Could you check a few things on this drawing? It's one solid part, dimensions in mm from its lowest x, y, z. Round coordinates to 2 decimals unless told otherwise and drop trailing zeros. Order: outer loops, then holes, each group sorted by start corner. A loop starts at its lowest first (then second) coordinate and runs counter-clockwise, first axis right, second up. Notation, with made-up numbers: (74, -12) - (79, -12) arc R27 ccw to (79, 6) - close; hole circle Ø1 at (61.5, 69.25). An arc over 180 degrees is marked (long way). Use one line per item in the form item = value.
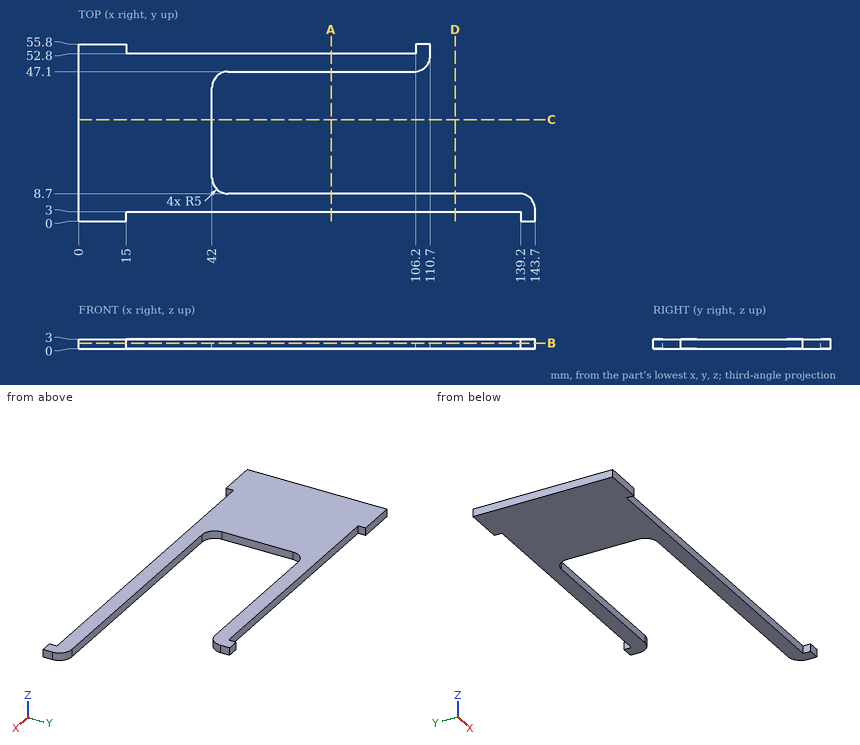
Item 1: Imagine slicing it at B-B on z = 1.8. Please give me the cut outline in (x, y), plus the area to 3 significant figures.
Found:
outline = (0, 0) - (15, 0) - (15, 3) - (139.2, 3) - (139.2, 0) - (143.7, 0) - (143.7, 3.7) arc R5 ccw to (138.7, 8.7) - (47, 8.7) arc R5 cw to (42, 13.7) - (42, 42.1) arc R5 cw to (47, 47.1) - (105.7, 47.1) arc R5 ccw to (110.7, 52.1) - (110.7, 55.8) - (106.2, 55.8) - (106.2, 52.8) - (15, 52.8) - (15, 55.8) - (0, 55.8) - close
area = 3,180 mm2
Item 2: Imagine slicing it at D-D on x = 118.5. Please give me the cut outline in (y, z).
Found:
outline = (3, 0) - (8.7, 0) - (8.7, 3) - (3, 3) - close
Item 3: Will these pins go through, and if not, where does the flat tip stop? P1, Ø0.9, axis at y = 53.5, z = 2, coming from the +X side; P2, Ø1, axis at y = 46, z = 2, coming from the +X side; P3, Ø1.5, axis at y = 7, z = 2.5, coming from the -X side; P4, Ø1.5, axis at x = 47, z = 1, coming from the -Y side.
Found:
P1 = 110.7
P2 = 44.63
P3 = 0
P4 = 3
Item 4: Imagine slicing it at C-C on y = 32. Please give me the cut outline in (x, z), plus the area to 3 significant figures.
Found:
outline = (0, 0) - (42, 0) - (42, 3) - (0, 3) - close
area = 126 mm2
Item 5: Imagine slicing it at A-A on x = 79.5. Please give me the cut outline in (y, z).
Found:
outline = (3, 0) - (8.7, 0) - (8.7, 3) - (3, 3) - close; (47.1, 0) - (52.8, 0) - (52.8, 3) - (47.1, 3) - close
Item 6: I need wall thicknesses on L1, parallel to Y at x = 102, z = 1.5; L2, parallel to Y at x = 120, z = 1.2; L3, parallel to X at y = 28, z = 0.75. Which ranges of each line are inside material? Lowest first, please.
Found:
L1 = 3 to 8.7, 47.1 to 52.8
L2 = 3 to 8.7
L3 = 0 to 42
